For this review, take the finished solid that the model builds, in its own axes (mm). A direction names the side the tool comes from. Round coordinates to 2 decimals unless told otherwise and drop trailing zeros. Write each loop counter-clockwise with the first axis right and the second up, starting at its lowest first coordinate (ties: lowest second). Pieces come first, ordered by that corner, then holes. Notation, with made-up numbers: (-32, 51.25) - (-20, 51.25) arc R26 cw to (-20, 66.25) - close; hole circle Ø11 at (84, 78). An arc over 180 degrees is marked (long way). One line per item, written item: value. Start each with the question number.
Q1. Clearance check with flat-ended pins moving along their axes: pin 1 Ø6 at (y, z) = (26, 29) entering from -X; pin 2 Ø10 at (x, y) = (-11, 88.5) entering from -Z; pin 3 Ø1.2 at (x, z) = (-16, 0.5) entering from -Y; pin 4 Ø3 at (x, y) = (-8, 71) entering from -Z. State where each tip first meets the part, or that it passes through.
Q2. Add section B-B on z = 10.5. Write out the cut boundary in (x, y), and give its area (3 significant figures).
Q3. Add section A-A on y = 20. Write out the cut boundary in (x, z), and give its area (3 significant figures).
Q4. Tool access review of faces 1 (the face through (-15.86, 75.9, 0.76)), 2 (the face through (0.86, 19.72, 0.9)), 3 (the face through (-8.923, 132.774, 0.739)): name each direction out of +Z, -Z, +X, -X, +Y, -Y from which nothing blocks a thin tool from reaching the whole face with its end or side.
Q5. Add section D-D on z = 34. Write out the cut boundary in (x, y), and give its area (3 significant figures).
Q6. Mouldability with a two-part tool opening along X and no side actions: class faces 4 (the face through (-8, 69, 1)), 5 (the face through (-24.1, 74.14, 0.76)), 6 (the face through (13.8, 6.3, 0.8)) as +X half, -X half, draft (parallel to the pull), parting line (faces both ways), or undercut.
Q7. For probe 1 along Y at (x, z) = (-23, 1.25); probe 2 along X at (y, z) = (131, 0.4); probe 3 along X at (y, z) = (35, 21.5), list the stretches that pass through material, from the lowest coordinate up.
Q8. Add section C-C on x = -13. Write out the cut boundary in (y, z), and give its area (3 significant figures).
```python
from build123d import *

# Parameters (mm, degrees)
BOSS_EXTRU_1_DEPTH           = 1.5
ENL_V_MAT_EXTRU_1_DEPTH      = 138.30349595
ESQUISSE3_W                  = 40
ESQUISSE3_H                  = 40
BOSS_EXTRU_2_DEPTH           = 1.5
ESQUISSE4_W                  = 4.5
ESQUISSE4_H                  = 2
ENL_V_MAT_EXTRU_2_DEPTH      = 1.5
ENL_V_MAT_EXTRU_5_DEPTH      = 144.003496461
CONG_1_R                     = 1
CONG_2_R                     = 3
ENL_V_MAT_EXTRU_3_DEPTH      = 144.699338899
ENL_V_MAT_EXTRU_3_DEPTH_BACK = 144.699338899
ESQUISSE9_R                  = 3.5
ENL_V_MAT_EXTRU_4_DEPTH      = 144.003496461
ENL_V_MAT_EXTRU_4_DEPTH_BACK = 144.003496461
ESQUISSE10_R                 = 2
CONVERTIR_VOLUME1_DEPTH      = 40
CONVERTIR_VOLUME1_2_DEPTH    = 40


# Read off the part's stored shape, not the designer's step: Convertir-Volume1
with BuildPart() as part:
    # Esquisse1 → Boss.-Extru.1 (new body)
    with BuildSketch(Plane.XY):
        Polygon((0, 0), (0, 47), (-8, 55), (-25, 55), (-25, 75), (-15, 75), (-15, 115), (-25, 115), (-25, 135), (0, 135), (0, 75.284271247), (20, 55.284271247), (20, 0), align=None)
    extrude(amount=BOSS_EXTRU_1_DEPTH)

    # Esquisse2 → Enlèv. mat.-Extru.1 (cut, through all)
    with BuildSketch(Plane.XY.offset(1.5)):
        with BuildLine():
            Line((-25, 69.582575695), (-25, 60.417424305))
            ThreePointArc((-25, 60.417424305), (-18, 65), (-25, 69.582575695))
        make_face()
        with BuildLine():
            Line((-25, 120.417424305), (-25, 129.582575695))
            ThreePointArc((-25, 129.582575695), (-18, 125), (-25, 120.417424305))
        make_face()
    extrude(amount=-ENL_V_MAT_EXTRU_1_DEPTH, mode=Mode.SUBTRACT)

    # Esquisse3 → Boss.-Extru.2 (add)
    with BuildSketch(Plane.ZY):
        with Locations((21.5, 20)):
            Rectangle(ESQUISSE3_W, ESQUISSE3_H)
    extrude(amount=-BOSS_EXTRU_2_DEPTH)

    # Esquisse4 → Enlèv. mat.-Extru.2 (cut)
    with BuildSketch(Plane.XY.offset(1.5)):
        with Locations((2.25, 41)):
            Rectangle(ESQUISSE4_W, ESQUISSE4_H)
    extrude(amount=-ENL_V_MAT_EXTRU_2_DEPTH, mode=Mode.SUBTRACT)

    # Esquisse11 → Enlèv. mat.-Extru.5 (cut, through all)
    with BuildSketch(Plane.XY.offset(1.5)):
        Polygon((20, 12.5), (7.5, 0), (20, 0), align=None)
    extrude(amount=-ENL_V_MAT_EXTRU_5_DEPTH, mode=Mode.SUBTRACT)

    # Congé1
    cong_1_edges = [part.edges().sort_by_distance(p)[0] for p in [
        (-25, 129.582575695, 0.75),
        (-25, 120.417424305, 0.75),
        (-25, 69.582575695, 0.75),
        (-25, 60.417424305, 0.75),
        (0, 42, 0.75),
        (4.5, 42, 0.75),
        (4.5, 40, 0.75),
    ]]
    fillet(cong_1_edges, radius=CONG_1_R - 0.0001)  # a hair under: the kernel refuses the full size

    # Congé2
    cong_2_edges = [part.edges().sort_by_distance(p)[0] for p in [
        (0, 47, 0.75),
        (-8, 55, 0.75),
        (-25, 55, 0.75),
        (-25, 75, 0.75),
        (-15, 75, 0.75),
        (-15, 115, 0.75),
        (-25, 115, 0.75),
        (-25, 135, 0.75),
        (0, 135, 0.75),
        (0, 75.284271247, 0.75),
        (20, 55.284271247, 0.75),
        (0.75, 40, 41.5),
        (0.75, 0, 41.5),
        (20, 12.5, 0.75),
        (7.5, 0, 0.75),
    ]]
    fillet(cong_2_edges, radius=CONG_2_R)

    # Esquisse9 → Enlèv. mat.-Extru.3 (cut, two sides: drawn at the far end of the back side and taken through both)
    with BuildSketch(Plane(origin=(1.5, 0, 0), x_dir=(0, 0, -1), z_dir=(1, 0, 0)).offset(-ENL_V_MAT_EXTRU_3_DEPTH_BACK)):
        with Locations((-34, 20)):
            Circle(ESQUISSE9_R)
        with Locations((-9, 20)):
            Circle(ESQUISSE9_R)
    extrude(amount=ENL_V_MAT_EXTRU_3_DEPTH + ENL_V_MAT_EXTRU_3_DEPTH_BACK, mode=Mode.SUBTRACT)

    # Esquisse10 → Enlèv. mat.-Extru.4 (cut, two sides: drawn at the far end of the back side and taken through both)
    with BuildSketch(Plane.XY.offset(1.5).offset(-ENL_V_MAT_EXTRU_4_DEPTH_BACK)):
        with Locations((-8, 59)):
            Circle(ESQUISSE10_R)
        with Locations(Location((-8, 71, 0), (0, 0, 180))):
            Circle(ESQUISSE10_R)
        with Locations((-8, 119)):
            Circle(ESQUISSE10_R)
        with Locations(Location((-8, 131, 0), (0, 0, 180))):
            Circle(ESQUISSE10_R)
    extrude(amount=ENL_V_MAT_EXTRU_4_DEPTH + ENL_V_MAT_EXTRU_4_DEPTH_BACK, mode=Mode.SUBTRACT)

    # Convertir-Volume1 outline → Convertir-Volume1 (cut)
    with BuildSketch(Plane(origin=(0, 0, 0), x_dir=(1, 0, 0), z_dir=(0, 1, 0))):
        with BuildLine():
            ThreePointArc((0, -3), (0.878679656, -0.878679656), (3, 0))
            Line((3, 0), (0, 0))
            Line((0, 0), (0, -3))
        make_face()
    extrude(amount=CONVERTIR_VOLUME1_DEPTH, mode=Mode.SUBTRACT)

    # Convertir-Volume1 2 outline → Convertir-Volume1 2 (add)
    with BuildSketch(Plane(origin=(0, 0, 0), x_dir=(1, 0, 0), z_dir=(0, 1, 0))):
        with BuildLine():
            Line((1.5, -1.5), (1.5, -3))
            ThreePointArc((1.5, -3), (1.939339828, -1.939339828), (3, -1.5))
            Line((3, -1.5), (1.5, -1.5))
        make_face()
    extrude(amount=CONVERTIR_VOLUME1_2_DEPTH)


solid = part.part
```
Result set:
1. pin 1: stops at x = 0
1. pin 2: stops at z = 0
1. pin 3: stops at y = 55
1. pin 4: passes through
2. outline: (0, 0) - (1.5, 0) - (1.5, 16.84) - (0, 16.84) - close; (0, 23.16) - (1.5, 23.16) - (1.5, 40) - (0, 40) - close
2. area: 50.5 mm^2
3. outline: (0, 3) arc R3 ccw to (3, 0) - (20, 0) - (20, 1.5) - (3, 1.5) arc R1.5 cw to (1.5, 3) - (1.5, 5.5) - (0, 5.5) - close; (0, 12.5) - (1.5, 12.5) - (1.5, 30.5) - (0, 30.5) - close; (0, 37.5) - (1.5, 37.5) - (1.5, 41.5) - (0, 41.5) - close
3. area: 67.6 mm^2
4. face 1: +Z, -Z, -X
4. face 2: -Z, -X, -Y
4. face 3: +Z, -Z
5. outline: (0, 0) - (1.5, 0) - (1.5, 16.5) - (0, 16.5) - close; (0, 23.5) - (1.5, 23.5) - (1.5, 40) - (0, 40) - close
5. area: 49.5 mm^2
6. face 4: undercut
6. face 5: -X half
6. face 6: +X half
7. probe 1: y = 55.17 to 60, 70 to 74.83, 115.17 to 120, 130 to 134.83
7. probe 2: x = -25 to -10, -6 to 0
7. probe 3: x = 0 to 1.5
8. outline: (55, 0) - (135, 0) - (135, 1.5) - (55, 1.5) - close
8. area: 120 mm^2
